Design review of the part built by this model. Coordinates are the model's own, in mm. Face numbers are marked on the shaded views. A direction names the side the tool comes from. Coordinates: 2 decimals unless noted, no trailing zeros. Write each loop counter-clockwise with the first axis right and the second up, starting at its lowest first coordinate (ties: lowest second). Pieces come first, ordered by that corner, then holes.
Q1. Machinability: for the marked faces 1, 2 and 3, which of the approach directions +Z, -Z, +X, -X, +Y, -Y give a long, thin tool a straight path to every point of the face, cutting with its end or side? Answer none if there is none.
Q2. Add section D-D, the plane x = -4. Give the boundary of the cut face in (y, z).
Q3. Clearance check with flat-ended pins moving along their axes: pin 1 Ø5.5 at (x, z) = (-1.5, -7) entering from +Y; pin 2 Ø1 at (y, z) = (2.5, 9.5) entering from -X; pin 3 Ø1 at (x, z) = (-21, 4.5) entering from -Y; pin 4 Ø1.5 at (y, z) = (14.5, 16.5) entering from -X. State where each tip first meets the part, or that it passes through.
Q4. Add section A-A, the plane z = 19. Give the boundary of the cut face in (x, y).
Q5. Add section C-C, the plane y = 5. Give the boundary of the cut face in (x, z).
Q6. Add section B-B, the plane x = -10.8. Give the boundary of the cut face in (y, z), plus the area to 3 significant figures.
Q7. To check wall thickness, follow probe 1 along Y at (x, z) = (-25, 9); probe 2 along Y at (x, z) = (-10.8, 21.65); probe 3 along Z at (x, y) = (11.5, 12). State the ranges of each line that lie inside material, in increasing order.
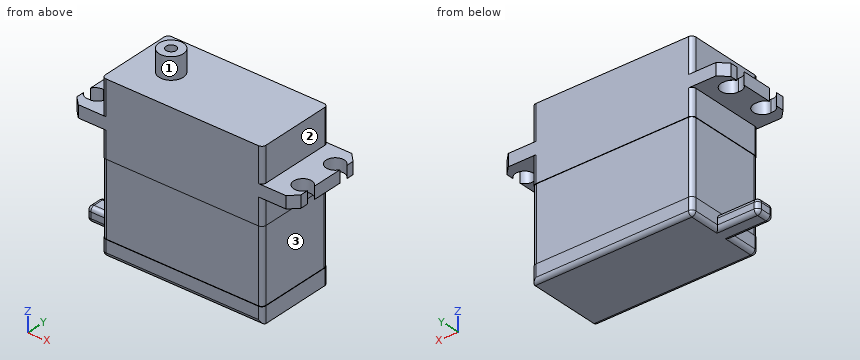
Autodesk Inventor part; units mm, degrees
ref_plane "Work Plane1" through (19.8, 0, 11.5) normal (0, 0, 1) x (1, 0, 0)
ref_plane "Work Plane2" through (0, 9.8, 0) normal (0, -1, 0) x (1, 0, 0)
ref_plane "YZ Plane" through (0, 0, 0) normal (1, 0, 0) x (0, 1, 0)
sketch "Sketch1" plane through (0, 0, 0) normal (0, 1, 0) x (-1, 0, 0)
  line L0 (-19.8, -20) -> (19.8, -20)
  line L1 (19.8, -20) -> (19.8, 20)
  line L2 (19.8, 20) -> (-19.8, 20)
  line L3 (-19.8, 20) -> (-19.8, -20)
  line L4 (-19.8, -20) -> (19.8, 20) construction
  line L5 (19.8, -20) -> (-19.8, 20) construction
  point P0 (0, 0)
  dimension "d0" = 39.6
  dimension "d1" = 40
extrude "Extrusion1" add sketch "Sketch1" along normal blind 19.6
sketch "Sketch2" plane through (-19.8, 0, -20) normal (-1, 0, 0) x (0, 0, 1)
  line L0 (31.5, 19.6) -> (28.5, 19.6)
  line L1 (28.5, 19.6) -> (28.5, 0)
  line L2 (28.5, 0) -> (31.5, 0)
  line L3 (31.5, 0) -> (31.5, 19.6)
  line L4 (0, 0) -> (0, 19.6)
  line L5 (0, 0) -> (40, 0)
  line L6 (0, 19.6) -> (40, 19.6)
  point P0 (20, 0)
  dimension "d4" = 28.5
  dimension "d5" = 3
  dimension "d6" = 0
  dimension "d7" = 0
extrude "Extrusion2" add sketch "Sketch2" along normal blind 7.8 contours L3 L2 L1 L0
sketch "Sketch4" plane through (-19.8, 0, 20) normal (0, 0, 1) x (1, 0, 0)
  circle A0 centre (9, 9.8) radius 3
  line L0 (0, 0) -> (39.6, 0)
  line L1 (0, 19.6) -> (39.6, 19.6)
  circle A1 centre (9, 9.8) radius 1.25
  line L2 (0, 0) -> (0, 19.6)
  line L3 (12, 3.6087) -> (12, 15.8306)
  point P0 (19.8, 0)
  dimension "d12" = 9.8
  dimension "d13" = 19.6
  dimension "d14" = 6
  dimension "d15" = 2.5
  dimension "d35" = 9
  dimension "d36" = 12
extrude "Extrusion4" add sketch "Sketch4" along normal blind 5.3
ref_plane "Work Plane1" through (19.8, 0, 11.5) normal (0, 0, 1) x (1, 0, 0)
sketch "Sketch5" plane through (19.8, 0, 11.5) normal (0, 0, 1) x (1, 0, 0)
  circle A0 centre (5.2, 5) radius 2.25
  line L0 (-47.4, 0) -> (-47.4, 19.7)
  line L1 (6.2685, 9.85) -> (-43.2578, 9.85)
  line L2 (-20.1, 2.75) -> (-20.1, 17.4196)
  circle A1 centre (5.2, 14.7) radius 2.25
  circle A2 centre (-45.4, 5) radius 2.25
  circle A3 centre (-45.4, 14.7) radius 2.25
  line L3 (0, 0) -> (0, 19.6)
  line L4 (-39.6, 0) -> (0, 0)
  point P0 (-19.8, 0)
  dimension "d18" = 4.5
  dimension "d41" = 5.2
  dimension "d42" = 5
  dimension "d43" = 9.7
extrude "Extrusion5" cut sketch "Sketch5" against normal blind 5
chamfer "Chamfer1" distance 2 angle 45 2 edges at (-27.6, 19.6, 10) (-27.6, 0, 10)
mirror "Mirror1" about plane through (0, 0, 0) normal (1, 0, 0) of "Extrusion2"
chamfer "Chamfer3" distance 2 angle 45 2 edges at (27.6, 19.6, 10) (27.6, 0, 10)
mirror "Mirror2" about plane through (0, 0, 0) normal (1, 0, 0) of "Extrusion5"
sketch "Sketch7" plane through (-19.8, 0, -20) normal (-1, 0, 0) x (0, 0, 1)
  line L0 (0, 0) -> (0, 19.6)
  line L1 (0, 12.1) -> (3.5, 12.1)
  line L2 (3.5, 12.1) -> (3.5, 7.6)
  line L3 (3.5, 7.6) -> (0, 7.6)
  line L4 (0, 7.6) -> (0, 12.1)
  line L5 (0, 0) -> (28.5, 0)
  line L6 (28.5, 19.7) -> (0, 19.7)
  line L7 (13.8096, 9.85) -> (-5.6461, 9.85) construction
  point P0 (20, 0)
  point P1 (0, 18.7)
  dimension "d44" = 4.5
  dimension "d45" = 19.7
  dimension "d46" = 9.85
  dimension "d47" = 3.5
extrude "Extrusion6" add sketch "Sketch7" along normal blind 10
sketch "Sketch8" plane through (0, 0, 0) normal (0, -1, 0) x (1, 0, 0)
  line L0 (-19.8, 2) -> (19.8, 2)
  line L1 (19.8, 2) -> (19.8, -16)
  line L2 (19.8, -16) -> (-19.8, -16)
  line L3 (-19.8, -16) -> (-19.8, 2)
  line L4 (19.8, -20) -> (-19.8, -20)
  line L5 (-19.8, -20) -> (-19.8, 8.5)
  line L6 (19.8, 8.5) -> (19.8, -20)
  point P0 (0, 0)
  dimension "d52" = 18
  dimension "d55" = 4
extrude "Extrusion7" cut sketch "Sketch8" against normal blind 0.1 contours L0 L1 L2 L3
ref_plane "Work Plane2" through (0, 9.8, 0) normal (0, -1, 0) x (1, 0, 0)
mirror "Mirror3" about plane through (0, 9.8, 0) normal (0, -1, 0) of "Extrusion7"
sketch "Sketch9" plane through (-19.8, 0, 8.5) normal (-1, 0, 0) x (0, 0, 1)
  line L0 (-6.5, 19.6) -> (-6.5, 19.5)
  line L1 (-24.5, 0.1) -> (-6.5, 0.1)
  line L2 (-6.5, 19.5) -> (-24.5, 19.5)
  line L3 (-24.5, 19.5) -> (-24.5, 0.1)
  line L4 (-24.5, 0.1) -> (-6.5, 0.1)
  line L5 (-6.5, 0.1) -> (-6.5, 19.5)
  point P0 (-8.5, 0)
extrude "Extrusion8" cut sketch "Sketch9" against normal blind 0.1
mirror "Mirror4" about plane through (0, 0, 0) normal (1, 0, 0) of "Extrusion8"
fillet "Fillet5" radius 1 28 edges at (-19.8, 0, 5.25) (-19.7, 0.1, -7) (-19.8, 0, 15.75) (-19.8, 0, -18) (-19.8, 3.8, -20) (0, 0, -20) (-19.8, 15.85, -20) (-24.8, 12.1, -16.5) (-24.8, 7.6, -16.5) (-24.8, 7.6, -20) (-29.8, 9.85, -20) (-29.8, 12.1, -18.25) (-24.8, 12.1, -20) (-29.8, 9.85, -16.5) (-29.8, 7.6, -18.25) (-19.8, 19.6, -18) (-19.7, 19.5, -7) (-19.8, 19.6, 5.25) (-19.8, 19.6, 15.75) (0, 19.6, -20) (19.8, 19.6, -18) (19.7, 19.5, -7) (19.8, 19.6, 5.25) (19.8, 19.6, 15.75) (19.8, 0, -18) (19.7, 0.1, -7) (19.8, 0, 5.25) (19.8, 0, 15.75)
equation "\"d12\" = 0.5 * d13"
equation "\"d46\" = 0.5 * d45"
properties part number "Trackstar_Servo_TS411MG"
Here are the results:
1. face 1: +Z
1. face 2: +Z, +X, +Y, -Y
1. face 3: +X, +Y, -Y
2. outline: (0, -19) arc R1 ccw to (1, -20) - (18.6, -20) arc R1 ccw to (19.6, -19) - (19.6, -16) - (19.5, -16) - (19.5, 2) - (19.6, 2) - (19.6, 20) - (0, 20) - (0, 2) - (0.1, 2) - (0.1, -16) - (0, -16) - close
3. pin 1: stops at y = 19.5
3. pin 2: stops at x = -27.6
3. pin 3: passes through
3. pin 4: stops at x = -19.8
4. outline: (-19.8, 1) arc R1 ccw to (-18.8, 0) - (18.8, 0) arc R1 ccw to (19.8, 1) - (19.8, 18.6) arc R1 ccw to (18.8, 19.6) - (-18.8, 19.6) arc R1 ccw to (-19.8, 18.6) - close
5. outline: (-22.75, 8.5) - (-19.8, 8.5) - (-19.8, 2) - (-19.7, 2) - (-19.7, -16) - (-19.8, -16) - (-19.8, -19) arc R1 ccw to (-18.8, -20) - (19.8, -20) - (19.8, -16) - (19.7, -16) - (19.7, 2) - (19.8, 2) - (19.8, 8.5) - (23.35, 8.5) - (23.35, 11.5) - (19.8, 11.5) - (19.8, 20) - (-19.8, 20) - (-19.8, 11.5) - (-22.75, 11.5) - close
6. outline: (0, -19) arc R1 ccw to (1, -20) - (18.6, -20) arc R1 ccw to (19.6, -19) - (19.6, -16) - (19.5, -16) - (19.5, 2) - (19.6, 2) - (19.6, 20) - (12.8, 20) - (12.8, 25.3) - (11.05, 25.3) - (11.05, 20) - (8.55, 20) - (8.55, 25.3) - (6.8, 25.3) - (6.8, 20) - (0, 20) - (0, 2) - (0.1, 2) - (0.1, -16) - (0, -16) - close
6. area: 799 mm2
7. probe 1: y = 0 to 2.75, 7.25 to 12.45, 16.95 to 19.6
7. probe 2: y = 6.8 to 8.55, 11.05 to 12.8
7. probe 3: z = -20 to 20
